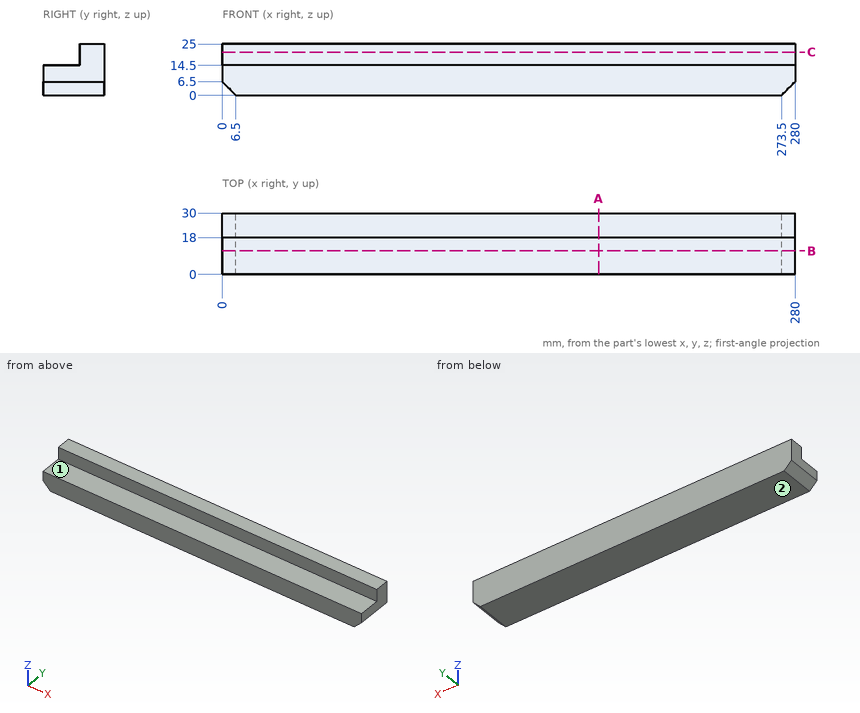
Geometry: see drawing. Coordinates: mm, zero at the bounding-box minimum. A direction names the side the tool comes from. Round coordinates to 2 decimals unless told otherwise and drop trailing zeros. Loops run counter-clockwise (first coordinate to the right, second up) from the corner with the lowest first, then second, coordinate; pieces in that order, holes last.
(1) Section query A-A (x = 184). Output: boundary loops of the cut face in (y, z), and give its area (3 significant figures).
From the geometry:
outline: (0, 0) - (30, 0) - (30, 25) - (18, 25) - (18, 14.5) - (0, 14.5) - close
area: 561 mm2
(2) Section query B-B (y = 11.5). Output: boundary loops of the cut face in (x, z), and give its area (3 significant figures).
From the geometry:
outline: (0, 6.5) - (6.5, 0) - (273.5, 0) - (280, 6.5) - (280, 14.5) - (0, 14.5) - close
area: 4,020 mm2
(3) Access query for the marked faces 1 and 2. Directions: +Z, -Z, +X, -X, +Y, -Y. A direction counts if a zero-diameter tool reaches every point of the face in a straight line with its end or side. Return the directions, or none.
From the geometry:
face 1: +Z, +X, -X, -Y
face 2: -Z, +X, -X, +Y, -Y
(4) Material intervals for probe 1 along Z at (x, y) = (42, 2.5); probe 2 along Y at (x, z) = (248, 17.5); probe 3 along X at (y, z) = (11.5, 1.5), sorted ascending.
From the geometry:
probe 1: z = 0 to 14.5
probe 2: y = 18 to 30
probe 3: x = 5 to 275
(5) Section query C-C (z = 21). Output: boundary loops of the cut face in (x, y).
From the geometry:
outline: (0, 18) - (280, 18) - (280, 30) - (0, 30) - close
(6) Contact query for a flat-ended pin moving along its axis: pin 1 Ø5 at (x, z) = (106, 18.5) entering from -Y. Output: stop coordinate, or through.
From the geometry:
pin 1: stops at y = 18
